Input: part model. Units: mm. Frame: model coordinates. Face numbers are marked on the shaded views. Round coordinates to 2 decimals unless told otherwise and drop trailing zeros. Order: outer loops, then holes, each group sorted by start corner. A loop starts at its lowest first (then second) coordinate and runs counter-clockwise, first axis right, second up. Notation, with made-up numbers: (24, -30) -> (68, -30) arc R21 cw to (68, 7) -> close; hole circle Ø11 at (-34, 2.25). An arc over 180 degrees is marked (long way). Use a Markdown table: item, result.
from build123d import *

# Parameters (mm, degrees)
SKETCH1_R           = 1.75
BOSS_EXTRUDE1_DEPTH = 3.175


with BuildPart() as part:
    # Sketch1 → Boss-Extrude1 (new body)
    with BuildSketch(Plane(origin=(0, 0, 0), x_dir=(1, 0, 0), z_dir=(0, 1, 0))):
        Polygon((-24.75, -3), (-24.75, 10), (-15, 10), (-15, 13.175), (-10, 13.175), (-10, 10), (10, 10), (10, 13.175), (15, 13.175), (15, 10), (24.75, 10), (24.75, -3), (19.6, -3), (19.6, 7), (-19.6, 7), (-19.6, -3), align=None)
        with Locations(Location((-21.85, 0, 0), (0, 0, 270))):
            Circle(SKETCH1_R, mode=Mode.SUBTRACT)
        with Locations(Location((21.85, 0, 0), (0, 0, 270))):
            Circle(SKETCH1_R, mode=Mode.SUBTRACT)
    extrude(amount=BOSS_EXTRUDE1_DEPTH)


solid = part.part
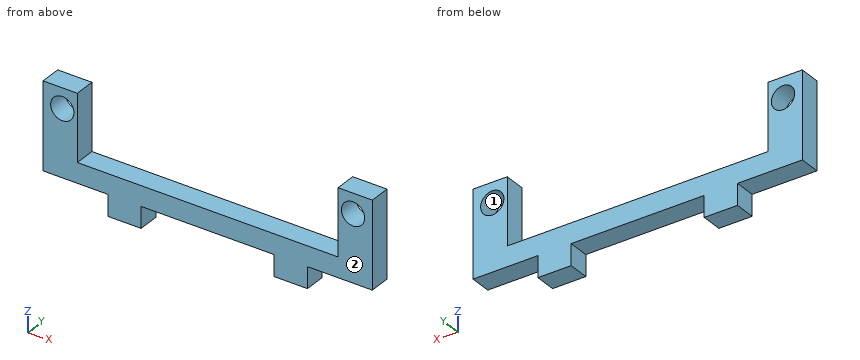
1) Line query: L1, parallel to X at y = 2.2, z = 0; L2, parallel to X at y = 1.85, z = 0.75; L3, parallel to Z at x = 22, y = 1.4. Output: solid intervals per line, ascending. Write a range as [from, to].
Results found:
| item | result |
|---|---|
| L1 | x = [-24.75, -23.6], [-20.1, -19.6], [19.6, 20.1], [23.6, 24.75] |
| L2 | x = [-24.75, -23.43], [-20.27, -19.6], [19.6, 20.27], [23.43, 24.75] |
| L3 | z = [-10, -1.74], [1.74, 3] |
2) Cut plane B-B on y = 2.75. Return loops of the section in (x, z) (3 decimals).
Results found:
| item | result |
|---|---|
| outline | (-24.75, -10) -> (-15, -10) -> (-15, -13.175) -> (-10, -13.175) -> (-10, -10) -> (10, -10) -> (10, -13.175) -> (15, -13.175) -> (15, -10) -> (24.75, -10) -> (24.75, 3) -> (19.6, 3) -> (19.6, -7) -> (-19.6, -7) -> (-19.6, 3) -> (-24.75, 3) -> close; hole circle Ø3.5 at (-21.85, 0); hole circle Ø3.5 at (21.85, 0) |
3) Pin query (flat end, axial travel): pin 1 Ø1.5 at (x, y) = (4, 2) entering from +Z; pin 2 Ø1 at (y, z) = (1.5, -11.5) entering from +X; pin 3 Ø1.5 at (x, y) = (5.5, 0.5) entering from -Z. Return the tip coordinate at first contact, or that it passes through.
Results found:
| item | result |
|---|---|
| pin 1 | stops at z = -7 |
| pin 2 | stops at x = 15 |
| pin 3 | stops at z = -10 |
4) Cut plane C-C on x = -21.85. Return loops of the section in (y, z) (3 decimals), and give its area (3 significant figures).
Results found:
| item | result |
|---|---|
| outline | (0, -10) -> (3.175, -10) -> (3.175, -1.75) -> (0, -1.75) -> close; (0, 1.75) -> (3.175, 1.75) -> (3.175, 3) -> (0, 3) -> close |
| area | 30.2 mm² |
5) Cut plane A-A on z = 0. Return loops of the section in (x, y) (3 decimals), and give its area (3 significant figures).
Results found:
| item | result |
|---|---|
| outline | (-24.75, 0) -> (-23.6, 0) -> (-23.6, 3.175) -> (-24.75, 3.175) -> close; (-20.1, 0) -> (-19.6, 0) -> (-19.6, 3.175) -> (-20.1, 3.175) -> close; (19.6, 0) -> (20.1, 0) -> (20.1, 3.175) -> (19.6, 3.175) -> close; (23.6, 0) -> (24.75, 0) -> (24.75, 3.175) -> (23.6, 3.175) -> close |
| area | 10.5 mm² |
6) Pull-direction query (Z, two-part tool) for the marked faces 1 and 2; classes: +Z half, -Z half, draft (parallel to the pull), parting line (faces both ways), or undercut.
Results found:
| item | result |
|---|---|
| face 1 | undercut |
| face 2 | draft |
7) Cut plane D-D on x = 6.5. Return loops of the section in (y, z) (3 decimals), and give its area (4 significant figures).
Results found:
| item | result |
|---|---|
| outline | (0, -10) -> (3.175, -10) -> (3.175, -7) -> (0, -7) -> close |
| area | 9.525 mm² |
